Build history of the part. All positions in model axes, mm. A direction names the side the tool comes from. Round coordinates to 2 decimals unless told otherwise and drop trailing zeros. Loops run counter-clockwise (first coordinate to the right, second up) from the corner with the lowest first, then second, coordinate; pieces in that order, holes last. Notation, with made-up numbers: M 68.5,28.5 L 87.5,28.5 A23 ccw 87.5,49.5 Z; hole C 16,-11.75 d10. An arc over 180 degrees is marked long. One line per item, written item: value.
```python
from build123d import *

# Parameters (mm, degrees)
SKETCH003_W     = 92
SKETCH003_H     = 61
PAD002_DEPTH    = 25
THICKNESS001_T  = 1
PAD003_DEPTH    = 61
SKETCH005_W     = 41
SKETCH005_H     = 25
POCKET001_DEPTH = 62


with BuildPart() as part:
    # Sketch003 → Pad002 (new body)
    with BuildSketch(Plane.XY):
        Rectangle(SKETCH003_W, SKETCH003_H)
    extrude(amount=PAD002_DEPTH)

    # Thickness001
    thickness001_openings = [part.faces().sort_by_distance(p)[0] for p in [
        (0, 0, 25),
    ]]
    offset(amount=THICKNESS001_T, openings=thickness001_openings)

    # Sketch004 (on DatumPlane) → Pad003 (join)
    with BuildSketch(Plane.XZ.offset(-30.5)):
        Polygon((46, 0), (-46, 0), (-46, 16), (-41, 16), (-41, 6), (-35, 6), (-35, 16), (-29, 16), (-29, 6), (-23, 6), (-23, 16), (-17, 16), (-17, 6), (-11, 6), (-11, 16), (-5, 16), (-5, 6), (1, 6), (1, 16), (7, 16), (7, 6), (13, 6), (13, 16), (18.287187, 16), align=None)
    extrude(amount=PAD003_DEPTH)

    # Sketch005 (on DatumPlane) → Pocket001 (cut)
    with BuildSketch(Plane.YZ.offset(-46)):
        with Locations((0, 12.5)):
            Rectangle(SKETCH005_W, SKETCH005_H)
    extrude(amount=POCKET001_DEPTH, mode=Mode.SUBTRACT)


solid = part.part
```
Item 1: Slice it at D-D, the plane z = 1. Give the cut face in (x, y).
Check values:
outline: M -47,-30.5 A1 ccw -46,-31.5 L 46,-31.5 A1 ccw 47,-30.5 L 47,30.5 A1 ccw 46,31.5 L -46,31.5 A1 ccw -47,30.5 Z; hole M -46,-20.5 L 16,-20.5 L 16,20.5 L -46,20.5 Z; hole M 44.27,-30.5 L 46,-30.5 L 46,30.5 L 44.27,30.5 Z
Item 2: Drop flat-ended pins along their axis: P1, Ø10, axis at x = -31, y = -1, coming from the +Z side; P2, Ø3, axis at x = -37.5, y = -23.5, coming from the +Z side; P3, Ø8, axis at x = 14, y = 23, coming from the +Z side. Give the stop position or say it passes through.
Check values:
P1: stops at z = 0
P2: stops at z = 6
P3: stops at z = 16
Item 3: Slice it at C-C, the plane x = -14. Give the cut face in (y, z), and give its area (3 significant figures).
Check values:
outline: M -31.5,0 A1 ccw -30.5,-1 L 30.5,-1 A1 ccw 31.5,0 L 31.5,25 L 30.5,25 L 30.5,6 L 20.5,6 L 20.5,0 L -20.5,0 L -20.5,6 L -30.5,6 L -30.5,25 L -31.5,25 Z
area: 233 mm2
Item 4: Which spindle directions (+Z, -Z, +X, -X, +Y, -Y) get a long thin tool onto all of the face, cutting with end or side? Do faces 1 (the face through (-20, -25, 16)), 2 (the face through (-47, 0, 12)). Say none if no direction does.
Check values:
face 1: +Z
face 2: +Z, -Z, -X, +Y, -Y
Item 5: Wall check: line 1 along X through (y, z) = (-26.5, 18.75); line 2 along Y through (x, z) = (-16.5, 9); line 3 along X through (y, z) = (-2, 15.25). Give the ranges that are in metal, low to high.
Check values:
line 1: x = -47 to -46, 46 to 47
line 2: y = -31.5 to -30.5, 30.5 to 31.5
line 3: x = -47 to -46, 16 to 19.59, 46 to 47
Item 6: Slice it at A-A, the plane z = 18. Give the cut face in (x, y), and give its area (3 significant figures).
Check values:
outline: M -47,-30.5 A1 ccw -46,-31.5 L 46,-31.5 A1 ccw 47,-30.5 L 47,30.5 A1 ccw 46,31.5 L -46,31.5 A1 ccw -47,30.5 Z; hole M -46,-30.5 L 46,-30.5 L 46,30.5 L -46,30.5 Z
area: 309 mm2
